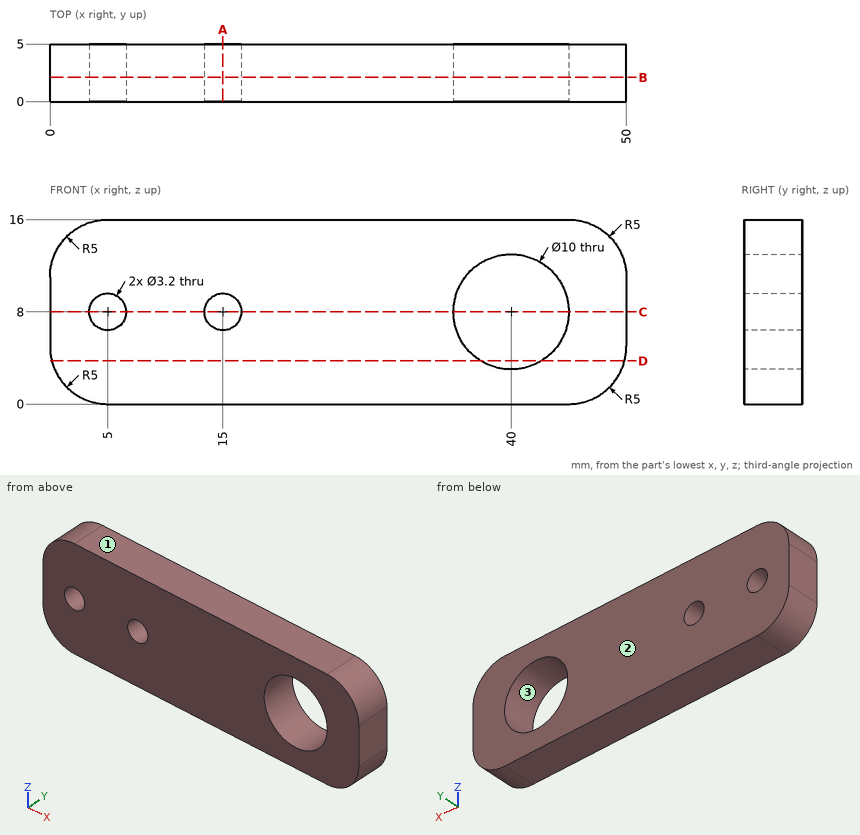
Study the drawing (mm; zero at the part's minimum x, y, z) and answer. Give positions to 0.01 mm unless a question says otherwise; leave off trailing zeros. Loops run counter-clockwise (first coordinate to the right, second up) from the corner with the lowest first, then second, coordinate; pieces in that order, holes last. Notation, with made-up numbers: (-40, -12) -> (1, -12) arc R14 cw to (1, 14) -> close; hole circle Ø11 at (37.25, -8.5). An arc over 180 degrees is marked (long way). Write item = value, one per line. Start each with the question number.
(1) Given pin 1 Ø1 at (y, z) = (4, 13) entering from +X, flat-ended and moving along its own axis, determine where the tip first touches the part or whether it passes through.
(2) Find the intervals of material crossed by probe 1 along X at (y, z) = (3.1, 8); probe 2 along X at (y, z) = (0.5, 11.25); probe 3 along Z at (x, y) = (42, 3.85), in increasing order. Write a range as from..to.
(3) Find section D-D on z = 3.75. Give the vertices of the cut face in (x, y).
(4) The mould has two halves that part along Z. Classify the marked faces 1, 2 and 3: +Z half, -Z half, draft (parallel to the pull), parting line (faces both ways), or undercut.
(5) Find section A-A on x = 15. Give the vertices of the cut face in (y, z).
(6) Find section C-C on z = 8. Give the vertices of the cut face in (x, y).
(7) Find section B-B on y = 2.1. Give the vertices of the cut face in (x, z), and give its area (3 significant figures).
From the geometry:
q1.pin_1 = 49.77
q2.probe_1 = 0..3.4, 6.6..13.4, 16.6..35, 45..50
q2.probe_2 = 0.01..36.2, 43.8..49.99
q2.probe_3 = 0..3.42, 12.58..16
q3.outline = (0.16, 0) -> (37.37, 0) -> (37.37, 5) -> (0.16, 5) -> close; (42.63, 0) -> (49.84, 0) -> (49.84, 5) -> (42.63, 5) -> close
q4.face_1 = +Z half
q4.face_2 = draft
q4.face_3 = undercut
q5.outline = (0, 0) -> (5, 0) -> (5, 6.4) -> (0, 6.4) -> close; (0, 9.6) -> (5, 9.6) -> (5, 16) -> (0, 16) -> close
q6.outline = (0, 0) -> (3.4, 0) -> (3.4, 5) -> (0, 5) -> close; (6.6, 0) -> (13.4, 0) -> (13.4, 5) -> (6.6, 5) -> close; (16.6, 0) -> (35, 0) -> (35, 5) -> (16.6, 5) -> close; (45, 0) -> (50, 0) -> (50, 5) -> (45, 5) -> close
q7.outline = (0, 5) arc R5 ccw to (5, 0) -> (45, 0) arc R5 ccw to (50, 5) -> (50, 11) arc R5 ccw to (45, 16) -> (5, 16) arc R5 ccw to (0, 11) -> close; hole circle Ø3.2 at (5, 8); hole circle Ø3.2 at (15, 8); hole circle Ø10 at (40, 8)
q7.area = 684 mm^2
